Part model, mm, in its own coordinate system. Coordinates: 2 decimals unless noted, no trailing zeros. Loops run counter-clockwise (first coordinate to the right, second up) from the corner with the lowest first, then second, coordinate; pieces in that order, holes last. Notation, with made-up numbers: (-27.75, -36.75) - (-23.75, -36.75) arc R33 cw to (-23.75, 1.25) - close; hole circle Ø6 at (69.25, -13). An arc over 180 degrees is marked (long way). Answer as CSV lines item,"result".
from build123d import *

# Parameters (mm, degrees)
F0_W     = 3.5
F0_H     = 20
F1_DEPTH = 3
F2_W     = 3
F2_H     = 20
F3_DEPTH = 3


with BuildPart() as f1:
    # F0 (on Top) → F1 (new body)
    with BuildSketch(Plane.XY):
        Polygon((60, 200), (60, 120), (0, 120), (0, 0), (400, 0), (400, 200), (240, 200), (240, 120), (180, 120), (180, 200), align=None)
        with Locations((228.25, 60)):
            Rectangle(F0_W, F0_H, mode=Mode.SUBTRACT)
    extrude(amount=F1_DEPTH)

    # F2 (on face) → F3 (join, through all)
    with BuildSketch(Plane.XY.offset(3)):
        with Locations((-1.5, 60)):
            Rectangle(F2_W, F2_H)
    extrude(amount=-F3_DEPTH)


solid = f1.part
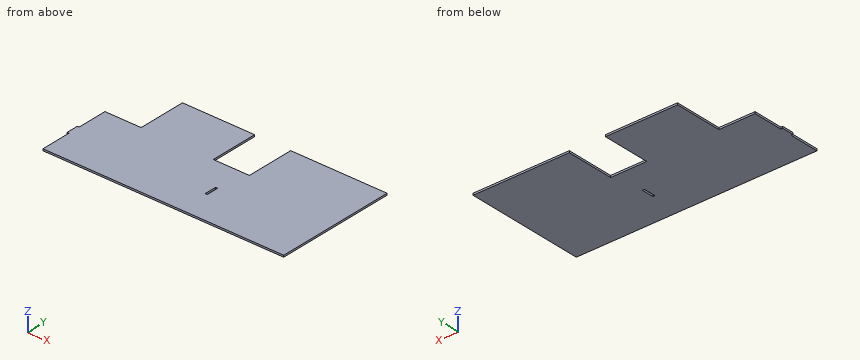
Q1. Flat gauge pins, fed straight in: pin 1 (0.9 mm diameter, centred on x = -1, z = 1, fed in from -Y); pin 2 (0.9 mm diameter, centred on y = 143, z = 1.5, fed in from -X); pin 3 (0.9 mm diameter, centred on x = 227.5, z = 1, fed in from +Y). Where does each tip first touch, or does it go through?
Results:
pin 1,"stops at y = 50"
pin 2,"stops at x = 60"
pin 3,"stops at y = 120"
Q2. Saw through at A-A (z = 2.35). Give the cut face in (x, y).
Results:
outline,"(-3, 50) - (0, 50) - (0, 0) - (400, 0) - (400, 200) - (240, 200) - (240, 120) - (180, 120) - (180, 200) - (60, 200) - (60, 120) - (0, 120) - (0, 70) - (-3, 70) - close; hole (226.5, 50) - (230, 50) - (230, 70) - (226.5, 70) - close"
Q3. Saw through at B-B (y = 154). Give the cut face in (x, z).
Results:
outline,"(60, 0) - (180, 0) - (180, 3) - (60, 3) - close; (240, 0) - (400, 0) - (400, 3) - (240, 3) - close"
Q4. Saw through at C-C (x = 55.5). Give the cut face in (y, z), then the cut area to 3 significant figures.
Results:
outline,"(0, 0) - (120, 0) - (120, 3) - (0, 3) - close"
area,"360 mm^2"
Q5. Wall check: L1, parallel to X at y = 152.5, z = 0.7; L2, parallel to X at y = 55, z = 0.45; L3, parallel to Y at x = 14.5, z = 1.65. Give the ranges that are in metal, low to high.
Results:
L1,"x = 60 to 180, 240 to 400"
L2,"x = -3 to 226.5, 230 to 400"
L3,"y = 0 to 120"
